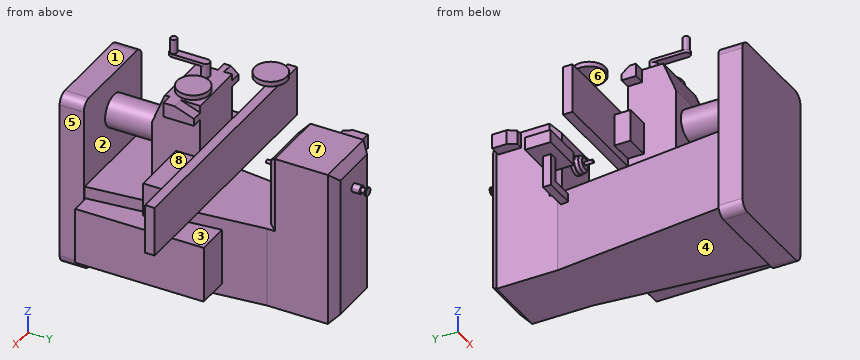
```python
from build123d import *

# Parameters (mm, degrees)
SKETCH_2_W          = 400
SKETCH_2_H          = 430
EXTRUDE_2_DEPTH     = 970
EXTRUDE_3_DEPTH     = 500
SKETCH_4_W          = 650
SKETCH_4_H          = 1100
EXTRUDE_4_DEPTH     = 150
SKETCH_5_R          = 25
EXTRUDE_5_DEPTH     = 50
SKETCH_6_R          = 15
EXTRUDE_6_DEPTH     = 30
SKETCH_7_R          = 25
EXTRUDE_7_DEPTH     = 10
CHAMFER_1_SIZE      = 50
SKETCH_8_R          = 55
EXTRUDE_8_DEPTH     = 20
SKETCH_9_R          = 50
EXTRUDE_9_DEPTH     = 40
CHAMFER_2_SIZE      = 15
SKETCH_10_R         = 10
EXTRUDE_10_DEPTH    = 50
SKETCH_11_W         = 360
SKETCH_11_H         = 300
EXTRUDE_11_DEPTH    = 660
SKETCH_12_W         = 1600
SKETCH_12_H         = 310
EXTRUDE_12_DEPTH    = 60
SKETCH_13_W         = 350
SKETCH_13_H         = 800
EXTRUDE_13_DEPTH    = 570
SKETCH_14_R         = 100
EXTRUDE_14_DEPTH    = 400
EXTRUDE_15_DEPTH    = 100
CUT_EXTRUDE_1_DEPTH = 10
SKETCH_17_R         = 100
EXTRUDE_16_DEPTH    = 30
CUT_EXTRUDE_2_REACH = 2181.284
SKETCH_19_W         = 370
SKETCH_19_H         = 210
EXTRUDE_17_DEPTH    = 150
SKETCH_20_W         = 150
SKETCH_20_H         = 200
EXTRUDE_18_DEPTH    = 100
SKETCH_21_R         = 25
EXTRUDE_19_DEPTH    = 70
SKETCH_22_R         = 100
EXTRUDE_20_DEPTH    = 30
EXTRUDE_21_DEPTH    = 20
SKETCH_24_R         = 20
EXTRUDE_22_DEPTH    = 90
SKETCH_25_W         = 80
SKETCH_25_H         = 90
EXTRUDE_23_DEPTH    = 70
CUT_EXTRUDE_3_DEPTH = 70
SKETCH_27_W         = 90
SKETCH_27_H         = 190
EXTRUDE_24_DEPTH    = 70
CUT_EXTRUDE_4_DEPTH = 70
FILLET_1_R          = 60
SKETCH_29_W         = 50
SKETCH_29_H         = 50
EXTRUDE_25_DEPTH    = 200
SKETCH_30_W         = 50
SKETCH_30_H         = 50
EXTRUDE_26_DEPTH    = 150
SKETCH_31_W         = 260
SKETCH_31_H         = 160
EXTRUDE_27_DEPTH    = 80


with BuildPart() as part:
    # ｽｹｯﾁ2 → ﾎﾞｽ - 押し出し2 (new body)
    with BuildSketch(Plane.XY):
        with Locations((136.676642933, -128.098797217)):
            Rectangle(SKETCH_2_W, SKETCH_2_H)
    extrude(amount=EXTRUDE_2_DEPTH)

    # ｽｹｯﾁ3 → ﾎﾞｽ - 押し出し3 (add)
    with BuildSketch(Plane(origin=(0, 0, 0), x_dir=(-1, 0, 0), z_dir=(0, 0, -1))):
        Polygon((-451.676642933, -1413.098797217), (178.323357067, -1413.098797217), (63.323357067, -343.098797217), (-336.676642933, -343.098797217), align=None)
    extrude(amount=-EXTRUDE_3_DEPTH)

    # ｽｹｯﾁ4 → ﾎﾞｽ - 押し出し4 (add)
    with BuildSketch(Plane(origin=(0, -1413.098797217, 0), x_dir=(-1, 0, 0), z_dir=(0, -1, 0))):
        with Locations((-136.676642933, -500)):
            Rectangle(SKETCH_4_W, SKETCH_4_H)
    extrude(amount=EXTRUDE_4_DEPTH)

    # ｽｹｯﾁ5 → ﾎﾞｽ - 押し出し5 (add)
    with BuildSketch(Plane(origin=(0, 86.901202783, 0), x_dir=(1, 0, 0), z_dir=(0, 1, 0))):
        with Locations(Location((136.676642933, -790, 0), (0, 0, 90))):
            Circle(SKETCH_5_R)
    extrude(amount=EXTRUDE_5_DEPTH)

    # ｽｹｯﾁ6 → ﾎﾞｽ - 押し出し6 (add)
    with BuildSketch(Plane(origin=(0, 136.901202783, 0), x_dir=(1, 0, 0), z_dir=(0, 1, 0))):
        with Locations(Location((136.676642933, -790, 0), (0, 0, 270))):
            Circle(SKETCH_6_R)
    extrude(amount=EXTRUDE_6_DEPTH)

    # ｽｹｯﾁ7 → ﾎﾞｽ - 押し出し7 (add)
    with BuildSketch(Plane(origin=(0, 166.901202783, 0), x_dir=(1, 0, 0), z_dir=(0, 1, 0))):
        with Locations(Location((136.676642933, -790, 0), (0, 0, 90))):
            Circle(SKETCH_7_R)
    extrude(amount=EXTRUDE_7_DEPTH)

    # 面取り1
    chamfer_1_edges = [part.edges().sort_by_distance(p)[0] for p in [
        (-63.323357067, 86.901202783, 485),
        (136.676642933, 86.901202783, 0),
        (136.676642933, 86.901202783, 970),
        (336.676642933, 86.901202783, 485),
        (-63.323357067, -343.098797217, 735),
        (336.676642933, -343.098797217, 735),
        (136.676642933, -343.098797217, 970),
    ]]
    chamfer(chamfer_1_edges, length=CHAMFER_1_SIZE)

    # ｽｹｯﾁ8 → ﾎﾞｽ - 押し出し8 (add)
    with BuildSketch(Plane(origin=(0, -343.098797217, 0), x_dir=(-1, 0, 0), z_dir=(0, -1, 0))):
        with Locations(Location((-136.676642933, -790, 0), (0, 0, 270))):
            Circle(SKETCH_8_R)
    extrude(amount=EXTRUDE_8_DEPTH)

    # ｽｹｯﾁ9 → ﾎﾞｽ - 押し出し9 (add)
    with BuildSketch(Plane(origin=(0, -363.098797217, 0), x_dir=(-1, 0, 0), z_dir=(0, -1, 0))):
        with Locations(Location((-136.676642933, -790, 0), (0, 0, 90))):
            Circle(SKETCH_9_R)
    extrude(amount=EXTRUDE_9_DEPTH)

    # 面取り2
    chamfer_2_edges = [part.edges().sort_by_distance(p)[0] for p in [
        (136.676642933, -403.098797217, 840),
    ]]
    chamfer(chamfer_2_edges, length=CHAMFER_2_SIZE)

    # ｽｹｯﾁ10 → ﾎﾞｽ - 押し出し10 (add)
    with BuildSketch(Plane(origin=(0, -403.098797217, 0), x_dir=(-1, 0, 0), z_dir=(0, -1, 0))):
        with Locations(Location((-136.676642933, -790, 0), (0, 0, 90))):
            Circle(SKETCH_10_R)
    extrude(amount=EXTRUDE_10_DEPTH)

    # ｽｹｯﾁ11 → ﾎﾞｽ - 押し出し11 (add)
    with BuildSketch(Plane.XY.offset(500)):
        with Locations((146.676642933, -913.098797217)):
            Rectangle(SKETCH_11_W, SKETCH_11_H)
    extrude(amount=EXTRUDE_11_DEPTH)

    # ｽｹｯﾁ12 → ﾎﾞｽ - 押し出し12 (add)
    with BuildSketch(Plane(origin=(0, -763.098797217, 0), x_dir=(1, 0, 0), z_dir=(0, 1, 0))):
        with Locations((146.676642933, -715)):
            Rectangle(SKETCH_12_W, SKETCH_12_H)
    extrude(amount=EXTRUDE_12_DEPTH)

    # ｽｹｯﾁ13 → ﾎﾞｽ - 押し出し13 (add)
    with BuildSketch(Plane(origin=(0, 0, 0), x_dir=(0, 0, -1), z_dir=(1, 0, 0))):
        with Locations((-250, -1006.142275478)):
            Rectangle(SKETCH_13_W, SKETCH_13_H)
    extrude(amount=EXTRUDE_13_DEPTH)

    # ｽｹｯﾁ14 → ﾎﾞｽ - 押し出し14 (add)
    with BuildSketch(Plane(origin=(0, -1413.098797217, 0), x_dir=(1, 0, 0), z_dir=(0, 1, 0))):
        with Locations(Location((121.676642933, -810, 0), (0, 0, 90))):
            Circle(SKETCH_14_R)
    extrude(amount=EXTRUDE_14_DEPTH)

    # ｽｹｯﾁ15 → ﾎﾞｽ - 押し出し15 (add)
    with BuildSketch(Plane.XY.offset(970)):
        Polygon((-63.323357067, 25.333856753), (-133.323357067, 25.333856753), (-133.323357067, -64.666143247), (-103.323357067, -114.666143247), (-63.323357067, -114.666143247), align=None)
    extrude(amount=-EXTRUDE_15_DEPTH)

    # ｽｹｯﾁ16 → ｶｯﾄ - 押し出し1 (cut)
    with BuildSketch(Plane.XY.offset(970)):
        Polygon((-63.323357067, 25.333856753), (-133.323357067, 25.333856753), (-133.323357067, -64.666143247), (-103.323357067, -114.666143247), (-63.323357067, -114.666143247), align=None)
    extrude(amount=-CUT_EXTRUDE_1_DEPTH, mode=Mode.SUBTRACT)

    # ｽｹｯﾁ17 → ﾎﾞｽ - 押し出し16 (add)
    with BuildSketch(Plane.XY.offset(870)):
        with Locations(Location((-503.323357067, -783.098797217, 0), (0, 0, 168.463040967))):
            Circle(SKETCH_17_R)
    extrude(amount=EXTRUDE_16_DEPTH)

    # ｽｹｯﾁ18 → ｶｯﾄ - 押し出し2 (cut, up to next)
    with BuildSketch(Plane.ZY.offset(33.323357067), mode=Mode.PRIVATE) as cut_extrude_2_sk1:
        Polygon((1160, -1063.098797217), (1160, -983.098797217), (960, -1063.098797217), align=None)
    cut_extrude_2_tool1 = extrude(cut_extrude_2_sk1.sketch, amount=-CUT_EXTRUDE_2_REACH, mode=Mode.PRIVATE) & part.part
    add(cut_extrude_2_tool1.solids().sort_by_distance((-33.323357, -1036.432131, 1093.333333))[0], mode=Mode.SUBTRACT)

    # ｽｹｯﾁ19 → ﾎﾞｽ - 押し出し17 (add)
    with BuildSketch(Plane(origin=(0, -763.098797217, 0), x_dir=(-1, 0, 0), z_dir=(0, -1, 0))):
        with Locations((-511.676642933, -715)):
            Rectangle(SKETCH_19_W, SKETCH_19_H)
    extrude(amount=EXTRUDE_17_DEPTH)

    # ｽｹｯﾁ20 → ﾎﾞｽ - 押し出し18 (add)
    with BuildSketch(Plane(origin=(0, -763.098797217, 0), x_dir=(-1, 0, 0), z_dir=(0, -1, 0))):
        with Locations((108.323357067, -710)):
            Rectangle(SKETCH_20_W, SKETCH_20_H)
    extrude(amount=EXTRUDE_18_DEPTH)

    # ｽｹｯﾁ21 → ﾎﾞｽ - 押し出し19 (add)
    with BuildSketch(Plane.XY.offset(1160)):
        with Locations((46.676642933, -883.098797217)):
            Circle(SKETCH_21_R)
    extrude(amount=EXTRUDE_19_DEPTH)

    # ｽｹｯﾁ22 → ﾎﾞｽ - 押し出し20 (add)
    with BuildSketch(Plane.XY.offset(1160)):
        with Locations((206.676642933, -873.098797217)):
            Circle(SKETCH_22_R)
    extrude(amount=EXTRUDE_20_DEPTH)

    # ｽｹｯﾁ23 → ﾎﾞｽ - 押し出し21 (add)
    with BuildSketch(Plane.XY.offset(1230)):
        with BuildLine():
            Line((21.676642933, -883.098797217), (21.676642933, -1083.098797217))
            ThreePointArc((21.676642933, -1083.098797217), (46.676642933, -1108.098797217), (71.676642933, -1083.098797217))
            Line((71.676642933, -1083.098797217), (71.676642933, -883.098797217))
            ThreePointArc((71.676642933, -883.098797217), (46.676642933, -858.098797217), (21.676642933, -883.098797217))
        make_face()
    extrude(amount=EXTRUDE_21_DEPTH)

    # ｽｹｯﾁ24 → ﾎﾞｽ - 押し出し22 (add)
    with BuildSketch(Plane.XY.offset(1250)):
        with Locations(Location((46.676642933, -1083.098797217, 0), (0, 0, 180))):
            Circle(SKETCH_24_R)
    extrude(amount=EXTRUDE_22_DEPTH)

    # ｽｹｯﾁ25 → ﾎﾞｽ - 押し出し23 (add)
    with BuildSketch(Plane.ZY.offset(33.323357067)):
        with Locations((1120, -808.098797217)):
            Rectangle(SKETCH_25_W, SKETCH_25_H)
    extrude(amount=EXTRUDE_23_DEPTH)

    # ｽｹｯﾁ26 → ｶｯﾄ - 押し出し3 (cut)
    with BuildSketch(Plane.ZY.offset(103.323357067)):
        Polygon((1160, -763.098797217), (1120, -763.098797217), (1160, -813.098797217), align=None)
    extrude(amount=-CUT_EXTRUDE_3_DEPTH, mode=Mode.SUBTRACT)

    # ｽｹｯﾁ27 → ﾎﾞｽ - 押し出し24 (add)
    with BuildSketch(Plane(origin=(326.676642933, 0, 0), x_dir=(0, 0, -1), z_dir=(1, 0, 0))):
        with Locations((-1115, -858.098797217)):
            Rectangle(SKETCH_27_W, SKETCH_27_H)
    extrude(amount=EXTRUDE_24_DEPTH)

    # ｽｹｯﾁ28 → ｶｯﾄ - 押し出し4 (cut)
    with BuildSketch(Plane(origin=(396.676642933, 0, 0), x_dir=(0, 0, -1), z_dir=(1, 0, 0))):
        Polygon((-1115, -763.098797217), (-1160, -883.098797217), (-1160, -763.098797217), align=None)
    extrude(amount=-CUT_EXTRUDE_4_DEPTH, mode=Mode.SUBTRACT)

    # ﾌｨﾚｯﾄ1
    fillet_1_edges = [part.edges().sort_by_distance(p)[0] for p in [
        (461.676642933, -1488.098797217, -50),
        (461.676642933, -1488.098797217, 1050),
        (-188.323357067, -1488.098797217, 1050),
        (-188.323357067, -1488.098797217, -50),
    ]]
    fillet(fillet_1_edges, radius=FILLET_1_R)

    # ｽｹｯﾁ29 → ﾎﾞｽ - 押し出し25 (add)
    with BuildSketch(Plane.ZY.offset(63.323357067)):
        with Locations((445, -388.098797217)):
            Rectangle(SKETCH_29_W, SKETCH_29_H)
    extrude(amount=EXTRUDE_25_DEPTH)

    # ｽｹｯﾁ30 → ﾎﾞｽ - 押し出し26 (add)
    with BuildSketch(Plane.XY.offset(470)):
        with Locations((-238.323357067, -388.098797217)):
            Rectangle(SKETCH_30_W, SKETCH_30_H)
    extrude(amount=EXTRUDE_26_DEPTH)

    # ｽｹｯﾁ31 → ﾎﾞｽ - 押し出し27 (add)
    with BuildSketch(Plane.XY.offset(620)):
        with Locations((-238.323357067, -388.098797217)):
            Rectangle(SKETCH_31_W, SKETCH_31_H)
    extrude(amount=EXTRUDE_27_DEPTH)


solid = part.part
```
Check sheet for the modelled part. Datum: model origin and axes. Units: mm. Face numbers are marked on the shaded views. A direction names the side the tool comes from. Coordinates: 2 decimals unless noted, no trailing zeros. Order: outer loops, then holes, each group sorted by start corner. A loop starts at its lowest first (then second) coordinate and runs counter-clockwise, first axis right, second up. Notation, with made-up numbers: (-31, 83.25) -> (17, 83.25) arc R20 cw to (17, 94.25) -> close; hole circle Ø10 at (-23.75, 81). An arc over 180 degrees is marked (long way). Write item = value, one per line. Start each with the question number.
1) Cross-section at B-B (z = 647.5). Enter the section's corners in (x, y), then the cut area to 3 significant figures.
2) Access from +Z, -Z, +X, -X, +Y, -Y to the whole of each face (thin tool, end or side, straight path). Record for the marked faces 5, 6, 7 and 8.
3) Material ranges on L1, parallel to Y at x = 53, z = 891.5; L2, parallel to Z at x = 66, y = -937.5; L3, parallel to X at y = -162.5, z = 774, recorded low to high.
4) Mould release check, pull along Z, two halves, no side actions. Record for the marked faces 1, 2, 3 and 4: +Z half, -Z half, draft (parallel to the pull), parting line (faces both ways), or undercut.
5) Cross-section at C-C (y = -1377.5). Enter the section's corners in (x, z).
6) Cross-section at D-D (z = 108.5). Enter the section's corners in (x, y).
7) Go/stop test with flat-tipped pins: P1, Ø21, axis at x = -94, z = 926, coming from the +Y side; P2, Ø6, axis at y = -1018, z = 148, coming from the +X side; P3, Ø2, axis at x = 116, z = 1099.5, coming from the -Y side. Record where each tip stops, or that it passes through.
8) Cross-section at A-A (x = -304). Enter the section's corners in (y, z), then the cut area to 3 significant figures.
Ans:
q1.outline = (-653.32, -763.1) -> (-183.32, -763.1) -> (-183.32, -863.1) -> (-33.32, -863.1) -> (-33.32, -1063.1) -> (326.68, -1063.1) -> (326.68, -913.1) -> (696.68, -913.1) -> (696.68, -763.1) -> (946.68, -763.1) -> (946.68, -703.1) -> (-653.32, -703.1) -> close; (-368.32, -468.1) -> (-108.32, -468.1) -> (-108.32, -308.1) -> (-368.32, -308.1) -> close; (-188.32, -1563.1) -> (461.68, -1563.1) -> (461.68, -1413.1) -> (-188.32, -1413.1) -> close; (-63.32, -293.1) -> (-13.32, -343.1) -> (286.68, -343.1) -> (336.68, -293.1) -> (336.68, 36.9) -> (286.68, 86.9) -> (-13.32, 86.9) -> (-63.32, 36.9) -> close
q1.area = 581,000 mm²
q2.face_5 = +Z, -Z, +X, -Y
q2.face_6 = -Z, -X, -Y
q2.face_7 = +Z, +X, -X, +Y
q2.face_8 = +X
q3.L1 = -1563.1 to -1413.1, -1063.1 to -763.1, -343.1 to 86.9
q3.L2 = 0 to 1160, 1230 to 1250
q3.L3 = -63.32 to 336.68
q4.face_1 = +Z half
q4.face_2 = undercut
q4.face_3 = undercut
q4.face_4 = -Z half
q5.outline = (-174.5, 0) -> (447.85, 0) -> (447.85, 75) -> (570, 75) -> (570, 425) -> (447.85, 425) -> (447.85, 500) -> (-174.5, 500) -> close; circle Ø200 at (121.68, 810)
q6.outline = (-188.32, -1563.1) -> (461.68, -1563.1) -> (461.68, -1413.1) -> (451.68, -1413.1) -> (450.93, -1406.14) -> (570, -1406.14) -> (570, -606.14) -> (364.95, -606.14) -> (336.68, -343.1) -> (336.68, 36.9) -> (286.68, 86.9) -> (-13.32, 86.9) -> (-63.32, 36.9) -> (-63.32, -343.1) -> (-178.32, -1413.1) -> (-188.32, -1413.1) -> close
q7.P1 = 25.33
q7.P2 = 570
q7.P3 = -1007.7
q8.outline = (-763.1, 560) -> (-703.1, 560) -> (-703.1, 870) -> (-763.1, 870) -> close; (-468.1, 620) -> (-308.1, 620) -> (-308.1, 700) -> (-468.1, 700) -> close
q8.area = 31,400 mm²
